Source: CAD feature listing. Evaluate the final solid. Frame: model axes, mm. Round coordinates to 2 decimals unless told otherwise and drop trailing zeros. Loops run counter-clockwise (first coordinate to the right, second up) from the corner with the lowest first, then second, coordinate; pieces in that order, holes last.
Item 1: First-contact query: P1, Ø20.5, axis at x = -127, y = 0, coming from the +Z side; P2, Ø12, axis at y = -9, z = -44.5, coming from the -X side. Flat tips, straight axial feed; report the tip coordinate or a pass-through.
Item 2: Ray query, L1, parallel to Y at x = -127, z = -86.9; L2, parallel to Z at x = -59, y = -14; L3, parallel to Y at x = 24, z = -34. Return the intervals inside material, ascending.
Item 3: Section query A-A on x = -127. Return loops of the section in (y, z).
Item 4: Section query C-C on x = -54. Return loops of the section in (y, z).
Item 5: Section query B-B on y = 15. Return loops of the section in (x, z), then the cut area to 3 significant figures.
Item 6: Pull-direction query (Y, two-part tool) for faces 1 (the cylindrical face through (-139.688, 0.558, -87.612)), 2 (the cylindrical face through (17.912, 6.867, -7.47)), 3 (the flat face through (-49, 0, -88.9)); classes: released by +Y, released by -Y, zero draft, split by the parting line, or undercut.
Item 7: Section query D-D on y = 0. Return loops of the section in (x, z), then the cut area to 3 significant figures.
```python
from build123d import *

# Parameters (mm, degrees)
BOSS_EXTRUDE1_DEPTH      = 76.2
BOSS_EXTRUDE1_DEPTH_BACK = 88.9
SKETCH4_R                = 10.16
SKETCH7_W                = 203.2
SKETCH7_H                = 60.96
BOSS_EXTRUDE2_DEPTH      = 2.54
SKETCH8_W                = 203.2
SKETCH8_H                = 60.96
BOSS_EXTRUDE3_DEPTH      = 2.54
SKETCH9_R                = 12.7
CUT_EXTRUDE1_DEPTH       = 227.74390929


with BuildPart() as part:
    # Sketch4 → Boss-Extrude1 (new, two sides: drawn at the far end of the back side and taken through both)
    with BuildSketch(Plane.XY.offset(-BOSS_EXTRUDE1_DEPTH_BACK)):
        with Locations((25.4, 0)):
            Circle(SKETCH4_R)
    extrude(amount=BOSS_EXTRUDE1_DEPTH + BOSS_EXTRUDE1_DEPTH_BACK)

    # Sketch7 → Boss-Extrude2 (add)
    with BuildSketch(Plane(origin=(0, 0, -88.9), x_dir=(-1, 0, 0), z_dir=(0, 0, -1))):
        with Locations((50.8, 0)):
            Rectangle(SKETCH7_W, SKETCH7_H)
    extrude(amount=-BOSS_EXTRUDE2_DEPTH)

    # Sketch8 → Boss-Extrude3 (add)
    with BuildSketch(Plane.XY.offset(76.2)):
        with Locations((-50.8, 0)):
            Rectangle(SKETCH8_W, SKETCH8_H)
    extrude(amount=-BOSS_EXTRUDE3_DEPTH)

    # Sketch9 → Cut-Extrude1 (cut, through all)
    with BuildSketch(Plane.XY.offset(76.2)):
        with Locations((-127, 0)):
            Circle(SKETCH9_R)
    extrude(amount=-CUT_EXTRUDE1_DEPTH, mode=Mode.SUBTRACT)


solid = part.part
```
Data:
1. P1: passes through
1. P2: stops at x = 15.69
2. L1: y = -30.48 to -12.7, 12.7 to 30.48
2. L2: z = -88.9 to -86.36, 73.66 to 76.2
2. L3: y = -10.06 to 10.06
3. outline: (-30.48, -88.9) - (-12.7, -88.9) - (-12.7, -86.36) - (-30.48, -86.36) - close; (-30.48, 73.66) - (-12.7, 73.66) - (-12.7, 76.2) - (-30.48, 76.2) - close; (12.7, -88.9) - (30.48, -88.9) - (30.48, -86.36) - (12.7, -86.36) - close; (12.7, 73.66) - (30.48, 73.66) - (30.48, 76.2) - (12.7, 76.2) - close
4. outline: (-30.48, -88.9) - (30.48, -88.9) - (30.48, -86.36) - (-30.48, -86.36) - close; (-30.48, 73.66) - (30.48, 73.66) - (30.48, 76.2) - (-30.48, 76.2) - close
5. outline: (-152.4, -88.9) - (50.8, -88.9) - (50.8, -86.36) - (-152.4, -86.36) - close; (-152.4, 73.66) - (50.8, 73.66) - (50.8, 76.2) - (-152.4, 76.2) - close
5. area: 1,030 mm2
6. face 1: undercut
6. face 2: split by the parting line
6. face 3: zero draft
7. outline: (-152.4, -88.9) - (-139.7, -88.9) - (-139.7, -86.36) - (-152.4, -86.36) - close; (-152.4, 73.66) - (-139.7, 73.66) - (-139.7, 76.2) - (-152.4, 76.2) - close; (-114.3, -88.9) - (50.8, -88.9) - (50.8, -86.36) - (35.56, -86.36) - (35.56, 73.66) - (50.8, 73.66) - (50.8, 76.2) - (-114.3, 76.2) - (-114.3, 73.66) - (15.24, 73.66) - (15.24, -86.36) - (-114.3, -86.36) - close
7. area: 4,150 mm2
